Read the model definition and answer for the solid it produces. Units are mm, in the model's axes. A direction names the side the tool comes from. Coordinates: 2 decimals unless noted, no trailing zeros. Order: outer loops, then holes, each group sorted by start corner. A loop starts at its lowest first (then second) coordinate and runs counter-clockwise, first axis right, second up. Notation, with made-up numbers: (80.5, 48.5) - (137.5, 48.5) arc R15 ccw to (137.5, 69.5) - close; hole circle Ø5 at (52, 10.5). An arc over 180 degrees is marked (long way). Answer as a JSON object with one key per item and string values. Group by question number.
from build123d import *

# Parameters (mm, degrees)
EXTRUDE1_DEPTH = 2.24
CHAMFER1_SIZE  = 0.4905


with BuildPart() as part:
    # Sketch1 → Revolve1 (revolve)
    with BuildSketch(Plane.XZ.offset(-28.4)):
        Polygon((-11, -2), (-16, -2), (-16, -10), (-13.5, -10), (-13.5, -4.8), (-11, -2.3), align=None)
    revolve(axis=Axis((-16, 28.4, -2), (0, 0, -1)))

    # Sketch2 → Extrude1 (cut)
    with BuildSketch(Plane.XY.offset(-2)):
        Polygon((-17.5, 29.266025404), (-17.5, 27.533974596), (-16, 26.667949192), (-14.5, 27.533974596), (-14.5, 29.266025404), (-16, 30.132050808), align=None)
    extrude(amount=-EXTRUDE1_DEPTH, mode=Mode.SUBTRACT)

    # Sketch3 → Cut-Revolve1 (revolve, cut)
    with BuildSketch(Plane.XZ.offset(-28.4)):
        Polygon((-14.5, -4.24), (-16, -4.24), (-16, -4.641923789), align=None)
    revolve(axis=Axis((-16, 28.4, -4.239975), (0, 0, -1)), mode=Mode.SUBTRACT)

    # Chamfer1
    chamfer1_edges = [part.edges().sort_by_distance(p)[0] for p in [
        (-18.5, 28.4, -10),
    ]]
    chamfer(chamfer1_edges, length=CHAMFER1_SIZE)


solid = part.part
1. A cutting plane is placed at B-B on z = -6.75. Write down the section's boundary in (x, y).
2. For faces 4 (the flat face through (-16, 28, -10)), 5 (the cylindrical face through (-18.5, 28.3, -7.1)), 6 (the flat face through (-15.26, 27.095, -3.104)), determine the directions among +Z, -Z, +X, -X, +Y, -Y from which every point of the face is accessible in a straight line to the end or side of a thin tool.
3. A cutting plane is placed at A-A on z = -3.5. Write down the section's boundary in (x, y).
4. For a pull along Y with two mould halves and no side action, classify faces 1 (the flat face through (-16.74, 29.705, -3.104)), 2 (the flat face through (-15, 27, -2)), 3 (the cylindrical face through (-11.23, 26.9, -2.15)) as pulls with the +Y half, pulls with the -Y half, needs draft (parallel to the pull), parting line crosses it, or undercut.
5. Straight lines are drawn through the part: L1, parallel to Y at x = -18, z = -7.25; L2, parallel to Z at x = -18.75, y = 29.75; L3, parallel to Y at x = -17.25, z = -2.75. For each, find the intervals that lie inside material, in ascending order.
6. Given pin 1 (0.6 mm diameter, centred on x = -15, y = 28, fed in from +Z); pin 2 (4 mm diameter, centred on x = -16.5, z = -7, fed in from +Y); pin 3 (3 mm diameter, centred on y = 27, z = -3.5, fed in from -X), each flat-ended and moving along its own axis, determine where each tip first touches the part or whether it passes through.
Derived:
{
 "1": {"outline": "circle Ø5 at (-16, 28.4)"},
 "2": {"face 4": "-Z, +X, -X, +Y, -Y", "face 5": "-Z", "face 6": "+Z"},
 "3": {"outline": "circle Ø7.6 at (-16, 28.4); hole (-17.5, 27.53) - (-16, 26.67) - (-14.5, 27.53) - (-14.5, 29.27) - (-16, 30.13) - (-17.5, 29.27) - close"},
 "4": {"face 1": "undercut", "face 2": "needs draft", "face 3": "parting line crosses it"},
 "5": {"L1": "y = 26.9 to 29.9", "L2": "z = -4.24 to -2", "L3": "y = 24.03 to 27.39, 29.41 to 32.77"},
 "6": {"pin 1": "stops at z = -4.27", "pin 2": "stops at y = 30.9", "pin 3": "stops at x = -20.97"}
}
